Model file for the job. Use its own axes, mm. Round coordinates to 2 decimals unless told otherwise and drop trailing zeros. Write each loop counter-clockwise with the first axis right and the second up, starting at its lowest first coordinate (ties: lowest second). Pieces come first, ordered by that corner, then holes. Notation, with made-up numbers: (49, 34.25) - (63, 34.25) arc R22 ccw to (63, 53.25) - close; hole circle Ø7 at (-8, -22). An arc over 180 degrees is marked (long way). Answer as a JSON object with one key per item and string values. Group by question number.
from build123d import *

# Parameters (mm, degrees)
SKETCH004_R        = 94
SKETCH004_R_2      = 86
PAD005_DEPTH       = 2
SKETCH005_R        = 2.5
POCKET001_DEPTH    = 5
POLARPATTERN_COUNT = 8


with BuildPart() as part:
    # Sketch004 (on ShapeBinder) → Pad005 (new body)
    with BuildSketch(Plane.XZ):
        Circle(SKETCH004_R)
        Circle(SKETCH004_R_2, mode=Mode.SUBTRACT)
    extrude(amount=PAD005_DEPTH)

    # Sketch005 (on Face4 of Pad005) → Pocket001 (cut)
    with BuildSketch(Plane.XZ.offset(2)):
        with Locations((90, 0)):
            Circle(SKETCH005_R)
    pocket001 = extrude(amount=-POCKET001_DEPTH, mode=Mode.SUBTRACT)

    # PolarPattern: Pocket001 ×8 about axis
    polarpattern_axis = Axis((0, -2, 0), (0, -1, 0))
    for i in range(1, POLARPATTERN_COUNT):
        add(pocket001.rotate(polarpattern_axis, i * 360 / POLARPATTERN_COUNT), mode=Mode.SUBTRACT)


solid = part.part
(1) Drill centre lines: line 1 (X direction, y = -1.25, z = -27.5); line 2 (Z direction, x = 51, y = -0.75); line 3 (X direction, y = -1.1, z = 80). Where is each one in solid material? Low to high. Write a range as from..to.
(2) Slice it at C-C (x = 72.5). Write the cut outline in (y, z), then the cut area to 3 significant figures.
(3) Slice it at D-D (y = -0.5). Count the separate pieces of the cut face and the enclosed holes in it, then the cut area to 3 significant figures.
(4) Slice it at B-B (z = 8). Write the cut outline in (x, y).
(5) Slice it at A-A (x = 0). Write the cut outline in (y, z).
(6) Pull direction Z, two halves, no side cores. Call faces 1 (the cylindrical face through (-11.195, -0.986, 85.268)), 2 (the cylindrical face through (89.659, -0.986, 28.235)), 3 (the flat face through (41, -2, -76)): pulls with the +Z half, pulls with the -Z half, needs draft (parallel to the pull), parting line crosses it, or undercut.
(7) Flat gauge pins, fed straight in: pin 1 (6 mm diameter, centred on x = 63.64, z = 63.64, fed in from -Y); pin 2 (4.5 mm diameter, centred on x = -90, z = 0, fed in from -Y). Where does each tip first touch, or does it go through?
Answer:
{
 "1": {"line 1": "-89.89..-81.48, 81.48..89.89", "line 2": "-78.96..-69.25, 69.25..78.96", "line 3": "-49.36..-31.56, 31.56..49.36"},
 "2": {"outline": "(-2, -59.83) - (0, -59.83) - (0, -46.26) - (-2, -46.26) - close; (-2, 46.26) - (0, 46.26) - (0, 59.83) - (-2, 59.83) - close", "area": "54.3 mm²"},
 "3": {"separate pieces": "1", "enclosed holes": "9", "area": "4,370 mm²"},
 "4": {"outline": "(-93.66, -2) - (-85.63, -2) - (-85.63, 0) - (-93.66, 0) - close; (85.63, -2) - (93.66, -2) - (93.66, 0) - (85.63, 0) - close"},
 "5": {"outline": "(-2, -94) - (0, -94) - (0, -92.5) - (-2, -92.5) - close; (-2, -87.5) - (0, -87.5) - (0, -86) - (-2, -86) - close; (-2, 86) - (0, 86) - (0, 87.5) - (-2, 87.5) - close; (-2, 92.5) - (0, 92.5) - (0, 94) - (-2, 94) - close"},
 "6": {"face 1": "undercut", "face 2": "parting line crosses it", "face 3": "needs draft"},
 "7": {"pin 1": "y = -2", "pin 2": "through"}
}
